The model under review builds one solid part; all positions refer to its coordinate system, in mm. A direction names the side the tool comes from. Round coordinates to 2 decimals unless told otherwise and drop trailing zeros. Loops run counter-clockwise (first coordinate to the right, second up) from the corner with the lowest first, then second, coordinate; pieces in that order, holes last. Notation, with made-up numbers: M -37,0.25 L 6,0.25 A14 ccw 6,14.25 Z; hole C 2,88.25 d1. An arc over 180 degrees is marked long. Answer as a JSON object with one key per item and string values. Group by question number.
Item 1: Insertion check: P1, Ø0.8, axis at y = 1.5, z = 2, coming from the +X side; P2, Ø0.5, axis at x = 19.5, y = 1.5, coming from the -Z side; P3, Ø0.5, axis at y = 1.5, z = 2.5, coming from the -X side. Each pin has a flat end and moves straight along its axis. Give the tip position at first contact, or say it passes through.
Item 2: Consider section B-B (y = 1.7). Give the boundary of the cut face in (x, z), and give its area (3 significant figures).
Item 3: Consider section C-C (x = -21). Give the boundary of the cut face in (y, z), and give its area (4 significant figures).
Item 4: Consider section A-A (z = -15.5). Give the boundary of the cut face in (x, y).
Item 5: Tool access review of faces 1 (the face through (-63.32, 1.49, -24.25)), 2 (the face through (-65.5, 0.49, -26.82)), 3 (the face through (63.25, 1.49, -24.32)): name each direction out of +Z, -Z, +X, -X, +Y, -Y from which nothing blocks a thin tool from reaching the whole face with its end or side.
Item 6: To check wall thickness, follow line 1 (X direction, y = 1.45, z = -9); line 2 (Z direction, x = 18, y = 1.8); line 3 (X direction, y = 1.6, z = -23). State the ranges of each line that lie inside material, in increasing order.
```python
from build123d import *

# Parameters (mm, degrees)
BOSS_EXTRUDE1_DEPTH = 2
BOSS_EXTRUDE2_DEPTH = 1


with BuildPart() as part:
    # Sketch1 → Boss-Extrude1 (new body)
    with BuildSketch(Plane(origin=(0, 0, 0), x_dir=(1, 0, 0), z_dir=(0, 1, 0))):
        with BuildLine():
            Line((-59.75, 25.75), (59.75, 25.75))
            ThreePointArc((59.75, 25.75), (63.285533906, 24.285533906), (64.75, 20.75))
            Line((64.75, 20.75), (64.75, -25.75))
            Line((64.75, -25.75), (-64.75, -25.75))
            Line((-64.75, -25.75), (-64.75, 20.75))
            ThreePointArc((-64.75, 20.75), (-63.285533906, 24.285533906), (-59.75, 25.75))
        make_face()
    extrude(amount=BOSS_EXTRUDE1_DEPTH)

    # Sketch2 → Boss-Extrude2 (add)
    with BuildSketch(Plane(origin=(0, 0, 0), x_dir=(1, 0, 0), z_dir=(0, 1, 0))):
        with BuildLine():
            Line((-67, -25.75), (67, -25.75))
            Line((67, -25.75), (67, 23.25))
            ThreePointArc((67, 23.25), (65.535533906, 26.785533906), (62, 28.25))
            Line((62, 28.25), (-62, 28.25))
            ThreePointArc((-62, 28.25), (-65.535533906, 26.785533906), (-67, 23.25))
            Line((-67, 23.25), (-67, -25.75))
        make_face()
    extrude(amount=BOSS_EXTRUDE2_DEPTH)


solid = part.part
```
Geometry results:
{
 "1": {"P1": "stops at x = 64.75", "P2": "stops at z = -25.75", "P3": "stops at x = -64.75"},
 "2": {"outline": "M -64.75,-20.75 A5 ccw -59.75,-25.75 L 59.75,-25.75 A5 ccw 64.75,-20.75 L 64.75,25.75 L -64.75,25.75 Z", "area": "6,660 mm^2"},
 "3": {"outline": "M 0,-28.25 L 1,-28.25 L 1,-25.75 L 2,-25.75 L 2,25.75 L 0,25.75 Z", "area": "105.5 mm^2"},
 "4": {"outline": "M -67,0 L 67,0 L 67,1 L 64.75,1 L 64.75,2 L -64.75,2 L -64.75,1 L -67,1 Z"},
 "5": {"face 1": "-Z, -X, +Y", "face 2": "-Z, -X, +Y, -Y", "face 3": "-Z, +X, +Y"},
 "6": {"line 1": "x = -64.75 to 64.75", "line 2": "z = -25.75 to 25.75", "line 3": "x = -64.22 to 64.22"}
}
